Geometry check sheet. Reference: the model listing, model coordinates, mm. A direction names the side the tool comes from. Round coordinates to 2 decimals unless told otherwise and drop trailing zeros. Write each loop counter-clockwise with the first axis right and the second up, starting at its lowest first coordinate (ties: lowest second). Pieces come first, ordered by that corner, then holes.
from build123d import *

# Parameters (mm, degrees)
SKETCH2_R           = 3.75
BOSS_EXTRUDE1_DEPTH = 3.5
SKETCH2_5_R         = 3.75
BOSS_EXTRUDE2_DEPTH = 200
SKETCH3_R           = 3
CUT_EXTRUDE1_DEPTH  = 201


with BuildPart() as part:
    # Sketch2 → Boss-Extrude1 (new body)
    with BuildSketch(Plane(origin=(0, 0, 0), x_dir=(1, 0, 0), z_dir=(0, 1, 0))):
        with BuildLine():
            ThreePointArc((15.427248621, 1.5), (0, 15.5), (-15.427248621, 1.5))
            Line((-15.427248621, 1.5), (-5.809475019, 1.5))
            ThreePointArc((-5.809475019, 1.5), (0, 6), (5.809475019, 1.5))
            Line((5.809475019, 1.5), (15.427248621, 1.5))
        make_face()
        with Locations((0, 11.125)):
            Circle(SKETCH2_R, mode=Mode.SUBTRACT)
        with Locations((0, 11.125)):
            Circle(SKETCH2_R)
    extrude(amount=BOSS_EXTRUDE1_DEPTH)

    # Sketch2_5 → Boss-Extrude2 (add)
    with BuildSketch(Plane(origin=(0, 0, 0), x_dir=(1, 0, 0), z_dir=(0, 1, 0))):
        with Locations((0, 11.125)):
            Circle(SKETCH2_5_R)
    extrude(amount=BOSS_EXTRUDE2_DEPTH)

    # Sketch3 → Cut-Extrude1 (cut, through all)
    with BuildSketch(Plane(origin=(0, 200, 0), x_dir=(1, 0, 0), z_dir=(0, 1, 0))):
        with Locations((0, 11.125)):
            Circle(SKETCH3_R)
    extrude(amount=-CUT_EXTRUDE1_DEPTH, mode=Mode.SUBTRACT)


solid = part.part
1. Section check B-B (z = -4.25). Record the cut outline in (x, y).
2. Depth check by flat-ended pin: pin 1 Ø1 at (x, z) = (-5, -7.5) entering from +Y; pin 2 Ø5 at (y, z) = (118, -6) entering from +X; pin 3 Ø8 at (x, y) = (0.5, 82.5) entering from -Z (3 decimals). Enter the tip coordinate at first touch or a pass-through.
3. Section check A-A (x = 0). Record the cut outline in (y, z) (3 decimals), plus the area to 3 significant figures.
4. Section check D-D (x = -12). Record the cut outline in (y, z), plus the area to 3 significant figures.
5. Access from +Z, -Z, +X, -X, +Y, -Y to the whole of each face (thin tool, end or side, straight path). Record for faces 1 (the face through (-0.65, 101.4, -8.196)), 2 (the face through (-0.488, 100.374, -14.843)).
6. Scan lines: line 1 along Z through (x, y) = (0, 148) (3 decimals); line 2 along Y through (x, z) = (6.5, -7.25); line 3 along X through (y, z) = (101, -11.5). Record each from-to range of solid material in increasing order.
7. Section check C-C (y = 137.5). Record the cut outline in (x, z) (3 decimals), plus the area to 3 significant figures.
Results below:
1. outline: (-14.91, 0) - (-4.24, 0) - (-4.24, 3.5) - (-14.91, 3.5) - close; (4.24, 0) - (14.91, 0) - (14.91, 3.5) - (4.24, 3.5) - close
2. pin 1: stops at y = 3.5
2. pin 2: stops at x = 2.68
2. pin 3: stops at z = -14.875
3. outline: (0, -15.5) - (3.5, -15.5) - (3.5, -14.875) - (200, -14.875) - (200, -14.125) - (0, -14.125) - close; (0, -8.125) - (200, -8.125) - (200, -7.375) - (3.5, -7.375) - (3.5, -6) - (0, -6) - close
3. area: 307 mm2
4. outline: (0, -9.81) - (3.5, -9.81) - (3.5, -1.5) - (0, -1.5) - close
4. area: 29.1 mm2
5. face 1: +Y, -Y
5. face 2: +Y
6. line 1: z = -14.875 to -14.125, -8.125 to -7.375
6. line 2: y = 0 to 3.5
6. line 3: x = -3.73 to -2.98, 2.98 to 3.73
7. outline: circle Ø7.5 at (0, -11.125); hole circle Ø6 at (0, -11.125)
7. area: 15.9 mm2
